```python
from build123d import *

# Parameters (mm, degrees)
F0_W     = 34
F0_H     = 8
F1_DEPTH = 1.6
F2_R     = 1
F3_DEPTH = 1.601


with BuildPart() as f1:
    # F0 (on Front) → F1 (new body)
    with BuildSketch(Plane.XZ):
        Rectangle(F0_W, F0_H)
    extrude(amount=F1_DEPTH)

    # F2 (on face) → F3 (cut, through all)
    with BuildSketch(Plane.XZ.offset(1.6)):
        with Locations((-15, 0)):
            Circle(F2_R)
        with Locations((15, 0)):
            Circle(F2_R)
    extrude(amount=-F3_DEPTH, mode=Mode.SUBTRACT)


solid = f1.part
```
Verification items for the finished model (mm, model axes). Round coordinates to 2 decimals unless told otherwise and drop trailing zeros. Order: outer loops, then holes, each group sorted by start corner. A loop starts at its lowest first (then second) coordinate and runs counter-clockwise, first axis right, second up.
1) Cross-section at B-B, the plane x = 15. Record the cut outline in (y, z), plus the area to 3 significant figures.
Geometry says:
outline: (-1.6, -4) - (0, -4) - (0, -1) - (-1.6, -1) - close; (-1.6, 1) - (0, 1) - (0, 4) - (-1.6, 4) - close
area: 9.60 mm2
2) Depth check by flat-ended pin: pin 1 (1.2 mm diameter, centred on x = -15, z = 0, fed in from -Y). Enter the tip coordinate at first touch or a pass-through.
Geometry says:
pin 1: passes through
3) Material ranges on line 1 (Z direction, x = 15, y = -0.75); line 2 (X direction, y = -0.9, z = -0.75), recorded low to high.
Geometry says:
line 1: z = -4 to -1, 1 to 4
line 2: x = -17 to -15.66, -14.34 to 14.34, 15.66 to 17
4) Cross-section at A-A, the plane z = 0. Record the cut outline in (x, y).
Geometry says:
outline: (-17, -1.6) - (-16, -1.6) - (-16, 0) - (-17, 0) - close; (-14, -1.6) - (14, -1.6) - (14, 0) - (-14, 0) - close; (16, -1.6) - (17, -1.6) - (17, 0) - (16, 0) - close
5) Cross-section at C-C, the plane y = -0.95. Record the cut outline in (x, z).
Geometry says:
outline: (-17, -4) - (17, -4) - (17, 4) - (-17, 4) - close; hole circle Ø2 at (-15, 0); hole circle Ø2 at (15, 0)
6) Draft check along X on faces 1 (the cylindrical face through (-14, -1, 0)), 2 (the flat face through (17, -1, 0)), 3 (the flat face through (0, -1.6, 0)). Enter one of: +X half, -X half, draft (parallel to the pull), parting line (faces both ways), or undercut.
Geometry says:
face 1: undercut
face 2: +X half
face 3: draft
